Could you check a few things on this model? Use its own coordinates, in mm. Coordinates: 2 decimals unless noted, no trailing zeros. Loops run counter-clockwise (first coordinate to the right, second up) from the corner with the lowest first, then second, coordinate; pieces in that order, holes last. Notation, with made-up numbers: (45.25, 41) -> (51.25, 41) arc R27 cw to (51.25, 68) -> close; hole circle Ø7 at (-5.75, -3). An arc over 180 degrees is marked (long way). One line per question, with ' | ' between items. Start each with the question number.
(1) Suppose I cut it at D-D (z = -5). Please give me the cut outline in (x, y).
(2) Suppose I cut it at B-B (x = -4). Please give me the cut outline in (y, z).
(3) I'm going to push flat-ended pins straight in: pin 1 Ø2.5 at (x, z) = (4, 0) entering from +Y; pin 2 Ø1 at (x, y) = (2, 0.5) entering from +Z. Where does each tip first touch, or does it pass through?
(4) If I drill on line 1 along X through (y, z) = (1.8, 0); line 2 along X through (y, z) = (1.15, 0); line 3 along Z through (x, y) = (-4, 1.95), over which ranges is the centre line in solid material (lowest first)?
(5) If we mould it in two halves opening along X, with no side actions, what happens to faces 1 (the face through (0, 2, 0)), 2 (the face through (-9.76, 0.99, -2.17)), 3 (the face through (-2.43, 1.64, 0.35))? For each: pulls with the +X half, pulls with the -X half, needs draft (parallel to the pull), parting line crosses it, or undercut.
(6) Suppose I cut it at C-C (y = 0.75). Please give me the cut outline in (x, z), plus the area to 3 significant figures.
(7) Suppose I cut it at A-A (z = 0). Please give me the cut outline in (x, y).
```python
from build123d import *

# Parameters (mm, degrees)
SKETCH_1_R               = 10
EXTRUDE_1_DEPTH          = 2
HOLE_WIZARD_2_AT_2_COUNT = 2
HOLE_WIZARD_2_AT_2_PITCH = 8


with BuildPart() as part:
    # 草图1 → 凸台-拉伸1 (new body)
    with BuildSketch(Plane(origin=(0, 0, 0), x_dir=(1, 0, 0), z_dir=(0, 1, 0))):
        with Locations(Location((0, 0, 0), (0, 0, 270))):
            Circle(SKETCH_1_R)
    extrude(amount=EXTRUDE_1_DEPTH)

    # 草图4 → 孔2 (revolve, cut)
    with BuildSketch(Plane(origin=(4, 0, 0), x_dir=(0, 0, -1), z_dir=(1, 0, 0))):
        Polygon((0, 0), (0, 2), (1.5, 2), (1.5, 1.75), (3.25, 0), align=None)
    hole_wizard_2 = revolve(axis=Axis((4, -6.445314094, 0), (0, 1, 0)), mode=Mode.SUBTRACT)

    # 孔2 at 2: 孔2 ×2
    with Locations(*[(-i * HOLE_WIZARD_2_AT_2_PITCH, 0, 0) for i in range(1, HOLE_WIZARD_2_AT_2_COUNT)]):
        add(hole_wizard_2, mode=Mode.SUBTRACT)


solid = part.part
```
Checks:
1) outline: (-8.66, 0) -> (8.66, 0) -> (8.66, 2) -> (-8.66, 2) -> close
2) outline: (0, -9.17) -> (2, -9.17) -> (2, -1.5) -> (1.75, -1.5) -> (0, -3.25) -> close; (0, 3.25) -> (1.75, 1.5) -> (2, 1.5) -> (2, 9.17) -> (0, 9.17) -> close
3) pin 1: passes through | pin 2: stops at z = 9.89
4) line 1: x = -10 to -5.5, -2.5 to 2.5, 5.5 to 10 | line 2: x = -10 to -6.1, -1.9 to 1.9, 6.1 to 10 | line 3: z = -9.17 to -1.5, 1.5 to 9.17
5) face 1: needs draft | face 2: parting line crosses it | face 3: undercut
6) outline: circle Ø20 at (0, 0); hole circle Ø5 at (-4, 0); hole circle Ø5 at (4, 0) | area: 275 mm^2
7) outline: (-10, 0) -> (-7.25, 0) -> (-5.5, 1.75) -> (-5.5, 2) -> (-10, 2) -> close; (-2.5, 1.75) -> (-0.75, 0) -> (0.75, 0) -> (2.5, 1.75) -> (2.5, 2) -> (-2.5, 2) -> close; (5.5, 1.75) -> (7.25, 0) -> (10, 0) -> (10, 2) -> (5.5, 2) -> close
